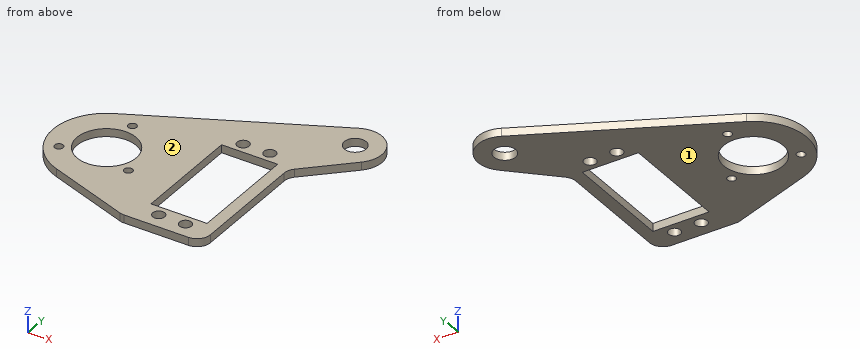
from build123d import *

# Parameters (mm, degrees)
SKETCH1_R               = 11.075
SKETCH1_R_2             = 4.075
BOSS_EXTRUDE1_DEPTH     = 3
CUT_EXTRUDE1_DEPTH      = 93.175105099
CUT_EXTRUDE1_DEPTH_BACK = 93.175105099
SKETCH2_R               = 1.575
CUT_EXTRUDE5_DEPTH      = 93.175105099
CUT_EXTRUDE5_DEPTH_BACK = 93.175105099
SKETCH6_R               = 2.25
FILLET2_R               = 5
CUT_EXTRUDE6_DEPTH      = 93.175105099
CUT_EXTRUDE6_DEPTH_BACK = 93.175105099
SKETCH7_W               = 21
SKETCH7_H               = 41


with BuildPart() as part:
    # Sketch1 → Boss-Extrude1 (new body)
    with BuildSketch(Plane.XY):
        with BuildLine():
            Line((24.96497351, -30), (-6.645635057, -18.863603439))
            ThreePointArc((-6.645635057, -18.863603439), (-19.962283564, -1.227694959), (-8.907060148, 17.907101371))
            Line((-8.907060148, 17.907101371), (60.546469926, 52.453550686))
            ThreePointArc((60.546469926, 52.453550686), (73.177271821, 49.256059899), (71.926246808, 36.28701829))
            Line((71.926246808, 36.28701829), (54.96497351, 20))
            Line((54.96497351, 20), (54.96497351, -30))
            Line((54.96497351, -30), (24.96497351, -30))
        make_face()
        Circle(SKETCH1_R, mode=Mode.SUBTRACT)
        with Locations((65, 43.5)):
            Circle(SKETCH1_R_2, mode=Mode.SUBTRACT)
    extrude(amount=BOSS_EXTRUDE1_DEPTH)

    # Sketch2 → Cut-Extrude1 (cut, two sides: drawn at the far end of the back side and taken through both)
    with BuildSketch(Plane.XY.offset(-CUT_EXTRUDE1_DEPTH_BACK)):
        with Locations((0, 15)):
            Circle(SKETCH2_R)
        with Locations((12.990381057, -7.5)):
            Circle(SKETCH2_R)
        with Locations((-12.990381057, -7.5)):
            Circle(SKETCH2_R)
    extrude(amount=CUT_EXTRUDE1_DEPTH + CUT_EXTRUDE1_DEPTH_BACK, mode=Mode.SUBTRACT)

    # Sketch6 → Cut-Extrude5 (cut, two sides: drawn at the far end of the back side and taken through both)
    with BuildSketch(Plane.XY.offset(-CUT_EXTRUDE5_DEPTH_BACK)):
        with Locations((35, -24)):
            Circle(SKETCH6_R)
        with Locations((35, 25)):
            Circle(SKETCH6_R)
        with Locations(Location((45, 25, 0), (0, 0, 180))):
            Circle(SKETCH6_R)
        with Locations(Location((45, -24, 0), (0, 0, 180))):
            Circle(SKETCH6_R)
    extrude(amount=CUT_EXTRUDE5_DEPTH + CUT_EXTRUDE5_DEPTH_BACK, mode=Mode.SUBTRACT)

    # Fillet2
    fillet2_edges = [part.edges().sort_by_distance(p)[0] for p in [
        (54.96497351, -30, 1.5),
        (24.96497351, -30, 1.5),
        (54.96497351, 20, 1.5),
    ]]
    fillet(fillet2_edges, radius=FILLET2_R)

    # Sketch7 → Cut-Extrude6 (cut, two sides: drawn at the far end of the back side and taken through both)
    with BuildSketch(Plane.XY.offset(-CUT_EXTRUDE6_DEPTH_BACK)):
        with Locations((40, 0.5)):
            Rectangle(SKETCH7_W, SKETCH7_H)
    extrude(amount=CUT_EXTRUDE6_DEPTH + CUT_EXTRUDE6_DEPTH_BACK, mode=Mode.SUBTRACT)


solid = part.part
Could you check a few things on this model? Use its own coordinates, in mm. Face numbers are marked on the shaded views. Give positions to 0.01 mm unless a question says otherwise; leave off trailing zeros. Loops run counter-clockwise (first coordinate to the right, second up) from the corner with the lowest first, then second, coordinate; pieces in that order, holes last. Notation, with made-up numbers: (-22.5, -40) -> (18.5, -40) arc R22 ccw to (18.5, -13) -> close; hole circle Ø1 at (-35, 24.25). An arc over 180 degrees is marked (long way). Return JSON: item names as keys, results as strings.
Item 1: If we section it at C-C on x = 65: List the corners of the cut face in (y, z) for me (3 decimals), plus the area to 3 significant figures.
Geometry results:
{"outline": "(29.636, 0) -> (39.425, 0) -> (39.425, 3) -> (29.636, 3) -> close; (47.575, 0) -> (53.5, 0) -> (53.5, 3) -> (47.575, 3) -> close", "area": "47.1 mm²"}
Item 2: I'm going to push flat-ended pins straight in: pin 1 (2.5 mm diameter, centred on x = 0, y = 15, fed in from -Z); pin 2 (0.9 mm diameter, centred on y = 10, z = 2, fed in from +X) (3 decimals); pin 3 (1 mm diameter, centred on x = 24.5, z = 1, fed in from -Y); pin 4 (0.9 mm diameter, centred on y = 1.5, z = 1.5, fed in from -X). Where does each tip first touch, or does it pass through?
Geometry results:
{"pin 1": "passes through", "pin 2": "stops at x = 54.965", "pin 3": "stops at y = -29.93", "pin 4": "stops at x = -19.97"}
Item 3: If we section it at B-B on z = 1.1: Count the separate pieces of the cut face and the enclosed holes in it, plus the area to 3 significant figures.
Geometry results:
{"separate pieces": "1", "enclosed holes": "10", "area": "3,210 mm²"}
Item 4: I need wall thicknesses on L1, parallel to Y at x = 45, z = 1.75; L2, parallel to X at y = -10, z = 2.3; L3, parallel to Y at x = 35.5, z = 1.8. Which ranges of each line are inside material? Lowest first, please. Write a range as from..to.
Geometry results:
{"L1": "y = -30..-26.25, -21.75..-20, 21..22.75, 27.25..44.72", "L2": "x = -17.32..-4.76, 4.76..29.5, 50.5..54.96", "L3": "y = -30..-26.19, -21.81..-20, 21..22.81, 27.19..40"}
Item 5: If we section it at D-D on y = 43.5: List the corners of the cut face in (x, z) for me (3 decimals).
Geometry results:
{"outline": "(42.546, 0) -> (60.925, 0) -> (60.925, 3) -> (42.546, 3) -> close; (69.075, 0) -> (75, 0) -> (75, 3) -> (69.075, 3) -> close"}
Item 6: If we section it at A-A on y = 0: List the corners of the cut face in (x, z) for me (3 decimals).
Geometry results:
{"outline": "(-20, 0) -> (-11.075, 0) -> (-11.075, 3) -> (-20, 3) -> close; (11.075, 0) -> (29.5, 0) -> (29.5, 3) -> (11.075, 3) -> close; (50.5, 0) -> (54.965, 0) -> (54.965, 3) -> (50.5, 3) -> close"}
Item 7: We'd pull the mould along Z, two halves only. Please class the marked faces 1 and 2: +Z half, -Z half, draft (parallel to the pull), parting line (faces both ways), or undercut.
Geometry results:
{"face 1": "-Z half", "face 2": "+Z half"}
